Source: CAD feature listing. Evaluate the final solid. Frame: model axes, mm. Give positions to 0.01 mm unless a question says otherwise; leave off trailing zeros. Order: outer loops, then holes, each group sorted by start corner. A loop starts at its lowest first (then second) coordinate and runs counter-clockwise, first axis right, second up. Notation, with made-up numbers: (-10, -11) - (23, -11) arc R30 ccw to (23, 13) - close; hole circle Ø2 at (87, 5). An arc over 180 degrees is marked (long way). One line per item, written item: value. Start each with the question number.
from build123d import *

# Parameters (mm, degrees)
F1_DEPTH = 6.35


with BuildPart() as f1:
    # F0 (on Top) → F1 (new body)
    with BuildSketch(Plane.XY):
        with BuildLine():
            ThreePointArc((-8.8427640474, 18.067783276), (-4.6419509437, 15.9641503371), (0, 15.24))
            ThreePointArc((0, 15.24), (4.6419509437, 15.9641503371), (8.8427640474, 18.067783276))
            ThreePointArc((8.8427640474, 18.067783276), (10.9985226281, 24.13), (15.1706770239, 29.0280500573))
            ThreePointArc((15.1706770239, 29.0280500573), (0, 45.72), (-15.1706770239, 29.0280500573))
            ThreePointArc((-15.1706770239, 29.0280500573), (-10.9985226281, 24.13), (-8.8427640474, 18.067783276))
        make_face()
        with BuildLine():
            ThreePointArc((11.049, 30.48), (7.8128228253, 22.6671771747), (0, 19.431))
            ThreePointArc((0, 19.431), (-7.8128228253, 38.2928228253), (11.049, 30.48))
        make_face(mode=Mode.SUBTRACT)
        with BuildLine():
            Line((0, 15.24), (0, 13.97))
            ThreePointArc((0, 13.97), (4.9605882744, 13.059611938), (9.2746396347, 10.4471029308))
            ThreePointArc((9.2746396347, 10.4471029308), (8.6449373915, 14.2339944405), (8.8427640474, 18.067783276))
            ThreePointArc((8.8427640474, 18.067783276), (4.6419509437, 15.9641503371), (0, 15.24))
        make_face()
        with BuildLine():
            ThreePointArc((-9.2746396347, 10.4471029308), (-4.9605882744, 13.059611938), (0, 13.97))
            Line((0, 13.97), (0, 15.24))
            ThreePointArc((0, 15.24), (-4.6419509437, 15.9641503371), (-8.8427640474, 18.067783276))
            ThreePointArc((-8.8427640474, 18.067783276), (-8.6449373915, 14.2339944405), (-9.2746396347, 10.4471029308))
        make_face()
        with BuildLine():
            ThreePointArc((0, -11.049), (-11.049, 0), (0, 11.049))
            Line((0, 11.049), (0, 13.97))
            ThreePointArc((0, 13.97), (-4.9605882744, 13.059611938), (-9.2746396347, 10.4471029308))
            ThreePointArc((-9.2746396347, 10.4471029308), (-10.9985226281, 6.35), (-13.6847763514, 2.8085220692))
            ThreePointArc((-13.6847763514, 2.8085220692), (-13.97, 0), (-13.6847763514, -2.8085220692))
            ThreePointArc((-13.6847763514, -2.8085220692), (-10.9985226281, -6.35), (-9.2746396347, -10.4471029308))
            ThreePointArc((-9.2746396347, -10.4471029308), (-4.9605882744, -13.059611938), (0, -13.97))
            Line((0, -13.97), (0, -11.049))
        make_face()
        with BuildLine():
            ThreePointArc((0, 11.049), (7.8128228253, 7.8128228253), (11.049, 0))
            ThreePointArc((11.049, 0), (7.8128228253, -7.8128228253), (0, -11.049))
            Line((0, -11.049), (0, -13.97))
            ThreePointArc((0, -13.97), (4.9605882744, -13.059611938), (9.2746396347, -10.4471029308))
            ThreePointArc((9.2746396347, -10.4471029308), (10.9985226281, -6.35), (13.6847763514, -2.8085220692))
            ThreePointArc((13.6847763514, -2.8085220692), (13.97, 0), (13.6847763514, 2.8085220692))
            ThreePointArc((13.6847763514, 2.8085220692), (10.9985226281, 6.35), (9.2746396347, 10.4471029308))
            ThreePointArc((9.2746396347, 10.4471029308), (4.9605882744, 13.059611938), (0, 13.97))
            Line((0, 13.97), (0, 11.049))
        make_face()
        with BuildLine():
            ThreePointArc((9.2746396347, -10.4471029308), (4.9605882744, -13.059611938), (0, -13.97))
            Line((0, -13.97), (0, -15.24))
            ThreePointArc((0, -15.24), (4.6419509437, -15.9641503371), (8.8427640474, -18.067783276))
            ThreePointArc((8.8427640474, -18.067783276), (8.6449373915, -14.2339944405), (9.2746396347, -10.4471029308))
        make_face()
        with BuildLine():
            Line((0, -15.24), (0, -13.97))
            ThreePointArc((0, -13.97), (-4.9605882744, -13.059611938), (-9.2746396347, -10.4471029308))
            ThreePointArc((-9.2746396347, -10.4471029308), (-8.6449373915, -14.2339944405), (-8.8427640474, -18.067783276))
            ThreePointArc((-8.8427640474, -18.067783276), (-4.6419509437, -15.9641503371), (0, -15.24))
        make_face()
        with BuildLine():
            ThreePointArc((8.8427640474, -18.067783276), (4.6419509437, -15.9641503371), (0, -15.24))
            ThreePointArc((0, -15.24), (-4.6419509437, -15.9641503371), (-8.8427640474, -18.067783276))
            ThreePointArc((-8.8427640474, -18.067783276), (-10.9985226281, -24.13), (-15.1706770239, -29.0280500573))
            ThreePointArc((-15.1706770239, -29.0280500573), (0, -45.72), (15.1706770239, -29.0280500573))
            ThreePointArc((15.1706770239, -29.0280500573), (10.9985226281, -24.13), (8.8427640474, -18.067783276))
        make_face()
        with BuildLine():
            ThreePointArc((11.049, -30.48), (-7.8128228253, -38.2928228253), (0, -19.431))
            ThreePointArc((0, -19.431), (7.8128228253, -22.6671771747), (11.049, -30.48))
        make_face(mode=Mode.SUBTRACT)
    extrude(amount=F1_DEPTH)


solid = f1.part
1. Ray query, L1, parallel to X at y = 31, z = 4; L2, parallel to Y at x = -2, z = 5; L3, parallel to Y at x = 8, z = 1.75. Return the intervals inside material, ascending.
2. Contact query for flat-ended pins moving along their axis: pin 1 Ø1 at (x, y) = (-9, -34) entering from -Z; pin 2 Ø2 at (y, z) = (3, 4) entering from +X. Output: stop coordinate, or through.
3. Section B-B on x = 3.5. Return the cut outline in (y, z).
4. Draft query along Y for faces 1 (the cylindrical face through (13.97, -0.04, 3.13)), 2 (the flat face through (-9, -7, 6.35)). Return one class per face: pulls with the +Y half, pulls with the -Y half, needs draft (parallel to the pull), parting line crosses it, or undercut.
5. Section D-D on x = 12. Return the cut outline in (y, z).
6. Section C-C on y = 35. Return the cut outline in (x, z).
7. Section A-A on z = 1. Return the cut outline in (x, y), then the cut area to 3 significant figures.
Data:
1. L1: x = -15.23 to -11.04, 11.04 to 15.23
1. L2: y = -45.59 to -41.35, -19.61 to -10.87, 10.87 to 19.61, 41.35 to 45.59
1. L3: y = -43.45 to -38.1, -22.86 to -7.62, 7.62 to 22.86, 38.1 to 43.45
2. pin 1: passes through
2. pin 2: stops at x = 13.83
3. outline: (-45.31, 0) - (-40.96, 0) - (-40.96, 6.35) - (-45.31, 6.35) - close; (-20, 0) - (-10.48, 0) - (-10.48, 6.35) - (-20, 6.35) - close; (10.48, 0) - (20, 0) - (20, 6.35) - (10.48, 6.35) - close; (40.96, 0) - (45.31, 0) - (45.31, 6.35) - (40.96, 6.35) - close
4. face 1: undercut
4. face 2: needs draft
5. outline: (-39.87, 0) - (-25.67, 0) - (-25.67, 6.35) - (-39.87, 6.35) - close; (-4.81, 0) - (4.81, 0) - (4.81, 6.35) - (-4.81, 6.35) - close; (25.67, 0) - (39.87, 0) - (39.87, 6.35) - (25.67, 6.35) - close
6. outline: (-14.55, 0) - (-10.08, 0) - (-10.08, 6.35) - (-14.55, 6.35) - close; (10.08, 0) - (14.55, 0) - (14.55, 6.35) - (10.08, 6.35) - close
7. outline: (-15.17, -29.03) arc R15.24 ccw (long way) to (15.17, -29.03) arc R17.78 cw to (13.68, -2.81) arc R13.97 ccw to (13.68, 2.81) arc R17.78 cw to (15.17, 29.03) arc R15.24 ccw (long way) to (-15.17, 29.03) arc R17.78 cw to (-13.68, 2.81) arc R13.97 ccw to (-13.68, -2.81) arc R17.78 cw to start; hole circle Ø22.1 at (0, -30.48); hole circle Ø22.1 at (0, 0); hole circle Ø22.1 at (0, 30.48)
7. area: 915 mm2
